Part model, mm, in its own coordinate system. Face numbers are marked on the shaded views. A direction names the side the tool comes from. Give positions to 0.01 mm unless a question says otherwise; leave off trailing zeros. Write each loop counter-clockwise with the first axis right and the second up, starting at its lowest first coordinate (ties: lowest second). Pieces come first, ordered by that corner, then holes. Notation, with made-up numbers: M 14.25,48 L 49.25,48 A17 cw 49.25,76 Z; hole C -40,49 d4. An arc over 180 degrees is marked long. Use a Markdown table: item, result.
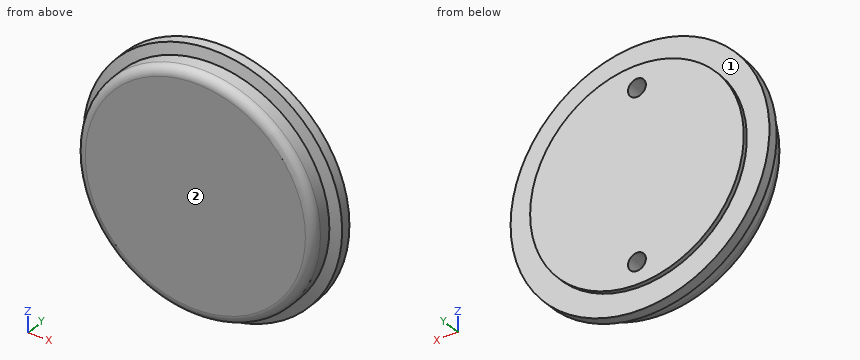
Autodesk Inventor part; units mm, degrees
ref_plane "YZ Plane" through (0, 0, 0) normal (1, 0, 0) x (0, 1, 0)
ref_plane "XZ Plane" through (0, 0, 0) normal (0, 1, 0) x (-1, 0, 0)
ref_plane "XY Plane" through (0, 0, 0) normal (0, 0, 1) x (1, 0, 0)
sketch "Sketch1" plane through (0, 0, 0) normal (0, 0, 1) x (1, 0, 0)
  line L0 (17.5514, 0) -> (46.0756, 0)
  line L1 (46.0756, 0) -> (46.0756, 12.7)
  line L2 (46.0756, 12.7) -> (0, 12.7)
  line L3 (0, 12.7) -> (0, 0)
  line L4 (17.5514, 12.7) -> (17.5514, 0)
  line L5 (46.0756, 8.9662) -> (42.3672, 8.9662)
  line L6 (42.3672, 7.747) -> (42.3672, 0)
  line L7 (46.0756, 7.747) -> (42.3672, 7.747)
  line L8 (46.0756, 8.9662) -> (42.3672, 7.747)
  line L9 (0, 11.1252) -> (0, 12.7)
  line L10 (17.5514, 0) -> (23.85, 0)
  line L11 (0, -2.5) -> (0, 0)
  line L12 (0, 12.7) -> (38.0365, 12.7)
  line L13 (38.0365, 12.7) -> (38.0365, 14.2748)
  line L14 (38.0365, 14.2748) -> (0, 14.2748)
  line L15 (0, 14.2748) -> (0, 12.7)
  line L16 (17.5514, 12.7) -> (17.5514, 14.2748)
  line L17 (0, 0) -> (17.5514, 0)
  dimension "d1" = 12.7
  dimension "d3" = 3.7338
  dimension "d5" = 4.953
  dimension "d8" = 17.5514
  dimension "d9" = 42.3672
  dimension "d10" = 46.0756
  dimension "d11" = 1.5748
  dimension "d12" = 38.0365
revolve "Revolution1" add sketch "Sketch1" angle 360 about axis through (0, 12.7, 0) along (0, -1, 0) contours L4 L2 L1 L8 L6 L0 | L17 L3 L2 L4 | L16 L14 L13 L2 | L2 L15 L14 L16
sketch "Sketch2" plane through (0, 14.2748, 0) normal (0, 1, 0) x (1, 0, 0)
  circle A0 centre (0, 0) radius 30.1752
  point P0 (0, 30.1752)
  point P1 (0, -30.1752)
  dimension "d14" = 60.3504
hole "Hole1" at (0, 14.2748, -30.1752) at (0, 14.2748, 30.1752) direction (0, -1, 0) diameter 6.35 depth 7.62
fillet "Fillet1" radius 3.175 1 edges at (-42.3672, 0, 0)
properties part number "2016.06.09 Blank Adapter" material "Aluminum 6061"
1. Tool access for the marked faces 1 and 2: list every direction of +Z, -Z, +X, -X, +Y, -Y with a clear straight run to the whole face (end or side of a thin tool).
Findings below:
| item | result |
|---|---|
| face 1 | +Y |
| face 2 | +Z, -Z, +X, -X, -Y |
2. Drill centre lines: L1, parallel to Z at x = 0, y = 11; L2, parallel to Z at x = -14, y = 9.75; L3, parallel to Y at x = 0, z = -32.5. Where is each one in solid material? Low to high.
Findings below:
| item | result |
|---|---|
| L1 | -46.08 to -33.35, -27 to 27, 33.35 to 46.08 |
| L2 | -43.9 to 43.9 |
| L3 | 0 to 6.65 |
3. Drop flat-ended pins along their axis: P1, Ø3, axis at y = 6, z = 15, coming from the -X side; P2, Ø10, axis at x = 0, z = -30.18, coming from the +Y side; P3, Ø5, axis at x = 0, z = 30.18, coming from the +Y side; P4, Ø2, axis at x = -31, y = 5.5, coming from the +Z side. Give the stop position or say it passes through.
Findings below:
| item | result |
|---|---|
| P1 | x = -40.16 |
| P2 | y = 14.27 |
| P3 | y = 6.65 |
| P4 | z = 29.92 |
4. Cut at A-A, the plane y = 11.25. Give the cut face in (x, z) (3 decimals).
Findings below:
| item | result |
|---|---|
| outline | C 0,0 d92.151; hole C 0,-30.175 d6.35; hole C 0,30.175 d6.35 |
